```python
from build123d import *

# Parameters (mm, degrees)
SKETCH1_W           = 81
SKETCH1_H           = 60
BOSS_EXTRUDE1_DEPTH = 2
SKETCH2_R           = 1.5
CUT_EXTRUDE1_DEPTH  = 51.440559077
FILLET1_R           = 4
CHAMFER1_SIZE       = 3
CHAMFER1_SIZE2      = 11.196152423
CHAMFER2_SIZE       = 3
CHAMFER2_SIZE2      = 11.196152423


with BuildPart() as part:
    # Sketch1 → Boss-Extrude1 (new body)
    with BuildSketch(Plane(origin=(0, 0, 0), x_dir=(1, 0, 0), z_dir=(0, 1, 0))):
        Rectangle(SKETCH1_W, SKETCH1_H)
    extrude(amount=BOSS_EXTRUDE1_DEPTH)

    # Sketch2 → Cut-Extrude1 (cut, through all)
    with BuildSketch(Plane(origin=(0, 2, 0), x_dir=(1, 0, 0), z_dir=(0, 1, 0))):
        with Locations(Location((-35.5, -25, 0), (0, 0, 270))):
            Circle(SKETCH2_R)
        with Locations(Location((35.5, -25, 0), (0, 0, 270))):
            Circle(SKETCH2_R)
        with Locations(Location((-35.5, 25, 0), (0, 0, 270))):
            Circle(SKETCH2_R)
        with Locations(Location((35.5, 25, 0), (0, 0, 270))):
            Circle(SKETCH2_R)
    extrude(amount=-CUT_EXTRUDE1_DEPTH, mode=Mode.SUBTRACT)

    # Fillet1
    fillet1_edges = [part.edges().sort_by_distance(p)[0] for p in [
        (-40.5, 1, -30),
        (40.5, 1, -30),
    ]]
    fillet(fillet1_edges, radius=FILLET1_R)

    # Chamfer1
    chamfer1_edges = [part.edges().sort_by_distance(p)[0] for p in [
        (40.5, 1, 30),
    ]]
    chamfer1_side = [part.faces().sort_by_distance(p)[0] for p in [
        (0, 1, 30),
    ]]
    chamfer(chamfer1_edges, length=CHAMFER1_SIZE, length2=CHAMFER1_SIZE2, reference=chamfer1_side[0])

    # Chamfer2
    chamfer2_edges = [part.edges().sort_by_distance(p)[0] for p in [
        (-40.5, 1, 30),
    ]]
    chamfer2_side = [part.faces().sort_by_distance(p)[0] for p in [
        (-1.5, 1, 30),
    ]]
    chamfer(chamfer2_edges, length=CHAMFER2_SIZE, length2=CHAMFER2_SIZE2, reference=chamfer2_side[0])


solid = part.part
```
Input: part model. Units: mm. Frame: model coordinates. Coordinates: 2 decimals unless noted, no trailing zeros. Write each loop counter-clockwise with the first axis right and the second up, starting at its lowest first coordinate (ties: lowest second). Pieces come first, ordered by that corner, then holes. Notation, with made-up numbers: (-34, 64) - (-15, 64) arc R20 cw to (-15, 81) - close; hole circle Ø5 at (22.25, -31). An arc over 180 degrees is marked (long way). Put each result on its own line as item: value. Start each with the question number.
1) Mould query, pull axis Z, two halves, no side actions, for faces 1 (the face through (-36.4, 1, -26.2)), 2 (the face through (-1, 1, 30)), 3 (the face through (-40.5, 1, -3)), 4 (the face through (39.297, 1.014, -28.859)). Classes: pulls with the +Z half, pulls with the -Z half, needs draft (parallel to the pull), parting line crosses it, or undercut.
2) Ray query, L1, parallel to X at y = 1.2, z = -25; L2, parallel to X at y = 1.25, z = -26; L3, parallel to X at y = 1.25, z = 22. Return the intervals inside material, ascending.
3) Cut plane B-B (z = -25). Return the cut outline in (x, y).
4) Cut plane A-A (x = 35.5). Return the cut outline in (y, z).
Resolved:
1. face 1: undercut
1. face 2: pulls with the +Z half
1. face 3: needs draft
1. face 4: pulls with the -Z half
2. L1: x = -40.5 to -37, -34 to 34, 37 to 40.5
2. L2: x = -40.5 to -36.62, -34.38 to 34.38, 36.62 to 40.5
2. L3: x = -39.64 to 39.64
3. outline: (-40.5, 0) - (-37, 0) - (-37, 2) - (-40.5, 2) - close; (-34, 0) - (34, 0) - (34, 2) - (-34, 2) - close; (37, 0) - (40.5, 0) - (40.5, 2) - (37, 2) - close
4. outline: (0, -30) - (2, -30) - (2, -26.5) - (0, -26.5) - close; (0, -23.5) - (2, -23.5) - (2, 23.5) - (0, 23.5) - close; (0, 26.5) - (2, 26.5) - (2, 30) - (0, 30) - close
